Design review of the part built by this model. Coordinates are the model's own, in mm. Face numbers are marked on the shaded views. A direction names the side the tool comes from. Round coordinates to 2 decimals unless told otherwise and drop trailing zeros. Order: outer loops, then holes, each group sorted by start corner. A loop starts at its lowest first (then second) coordinate and runs counter-clockwise, first axis right, second up.
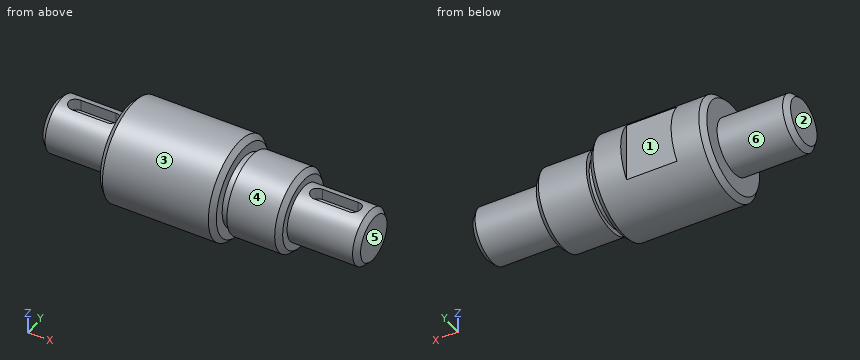
from build123d import *

# Parameters (mm, degrees)
SKETCH1_R               = 20
BOSS_EXTRUDE1_DEPTH     = 126
SKETCH2_OUTSIDE_W       = 69.624
SKETCH2_OUTSIDE_H       = 69.624
SKETCH2_OUTSIDE_R       = 11
CUT_EXTRUDE1_DEPTH      = 28
SKETCH3_OUTSIDE_W       = 69.624
SKETCH3_OUTSIDE_H       = 69.624
SKETCH3_OUTSIDE_R       = 11
CUT_EXTRUDE2_DEPTH      = 28
SKETCH4_OUTSIDE_W       = 69.624
SKETCH4_OUTSIDE_H       = 69.624
SKETCH4_OUTSIDE_R       = 16
CUT_EXTRUDE3_DEPTH      = 21
SKETCH5_OUTSIDE_W       = 69.624
SKETCH5_OUTSIDE_H       = 69.624
SKETCH5_OUTSIDE_R       = 14
CUT_EXTRUDE4_DEPTH      = 3
CHAMFER1_SIZE           = 2
CUT_EXTRUDE5_DEPTH      = 130.135587659
CUT_EXTRUDE5_DEPTH_BACK = 130.135587659
SKETCH6_W               = 20
SKETCH6_H               = 6
CUT_EXTRUDE6_DEPTH      = 5


with BuildPart() as part:
    # Sketch1 → Boss-Extrude1 (new body)
    with BuildSketch(Plane(origin=(0, 0, 0), x_dir=(0, 0, -1), z_dir=(1, 0, 0))):
        Circle(SKETCH1_R)
    extrude(amount=BOSS_EXTRUDE1_DEPTH)

    # Sketch2 outside → Cut-Extrude1 (cut)
    with BuildSketch(Plane.ZY):
        Rectangle(SKETCH2_OUTSIDE_W, SKETCH2_OUTSIDE_H)
        Circle(SKETCH2_OUTSIDE_R, mode=Mode.SUBTRACT)
    extrude(amount=-CUT_EXTRUDE1_DEPTH, mode=Mode.SUBTRACT)

    # Sketch3 outside → Cut-Extrude2 (cut)
    with BuildSketch(Plane(origin=(126, 0, 0), x_dir=(0, 0, -1), z_dir=(1, 0, 0))):
        Rectangle(SKETCH3_OUTSIDE_W, SKETCH3_OUTSIDE_H)
        with Locations(Location((0, 0, 0), (0, 0, 180))):
            Circle(SKETCH3_OUTSIDE_R, mode=Mode.SUBTRACT)
    extrude(amount=-CUT_EXTRUDE2_DEPTH, mode=Mode.SUBTRACT)

    # Sketch4 outside → Cut-Extrude3 (cut)
    with BuildSketch(Plane(origin=(98, 0, 0), x_dir=(0, 0, -1), z_dir=(1, 0, 0))):
        Rectangle(SKETCH4_OUTSIDE_W, SKETCH4_OUTSIDE_H)
        Circle(SKETCH4_OUTSIDE_R, mode=Mode.SUBTRACT)
    extrude(amount=-CUT_EXTRUDE3_DEPTH, mode=Mode.SUBTRACT)

    # Sketch5 outside → Cut-Extrude4 (cut)
    with BuildSketch(Plane(origin=(77, 0, 0), x_dir=(0, 0, -1), z_dir=(1, 0, 0))):
        Rectangle(SKETCH5_OUTSIDE_W, SKETCH5_OUTSIDE_H)
        Circle(SKETCH5_OUTSIDE_R, mode=Mode.SUBTRACT)
    extrude(amount=-CUT_EXTRUDE4_DEPTH, mode=Mode.SUBTRACT)

    # Chamfer1
    chamfer1_edges = [part.edges().sort_by_distance(p)[0] for p in [
        (0, 0, -11),
        (126, 0, -11),
        (98, 0, 16),
        (74, 0, 20),
        (28, 0, 20),
    ]]
    chamfer(chamfer1_edges, length=CHAMFER1_SIZE)

    # Sketch6 → Cut-Extrude5 (cut, two sides: drawn at the far end of the back side and taken through both)
    with BuildSketch(Plane.XY.offset(-CUT_EXTRUDE5_DEPTH_BACK)):
        with Locations((51, 19)):
            Rectangle(SKETCH6_W, SKETCH6_H)
    extrude(amount=CUT_EXTRUDE5_DEPTH + CUT_EXTRUDE5_DEPTH_BACK, mode=Mode.SUBTRACT)

    # Sketch7 → Cut-Extrude6 (cut)
    with BuildSketch(Plane.XY.offset(11)):
        with BuildLine():
            Line((8, 3), (22, 3))
            ThreePointArc((22, 3), (25, 0), (22, -3))
            Line((22, -3), (8, -3))
            ThreePointArc((8, -3), (5, 0), (8, 3))
        make_face()
        with BuildLine():
            Line((104, 3), (118, 3))
            ThreePointArc((118, 3), (121, 0), (118, -3))
            Line((118, -3), (104, -3))
            ThreePointArc((104, -3), (101, 0), (104, 3))
        make_face()
    extrude(amount=-CUT_EXTRUDE6_DEPTH, mode=Mode.SUBTRACT)


solid = part.part
1) To check wall thickness, follow line 1 along X through (y, z) = (-7, -9); line 2 along Y through (x, z) = (81, -0.5); line 3 along X through (y, z) = (17.5, 0). State the ranges of each line that lie inside material, in increasing order.
Results:
line 1: x = 28 to 98
line 2: y = -15.99 to 15.99
line 3: x = 28 to 41, 61 to 74
2) Take a section at C-C on x = 54. Give the boundary of the cut face in (y, z), plus the area to 3 significant figures.
Results:
outline: (16, -12) - (16, 12) arc R20 ccw (long way) to start
area: 1,190 mm2
3) The part is to be moulded in two halves that separate along X. For the marked faces 1, 2 and 3, say which applies: released by +X, released by -X, zero draft, split by the parting line, or undercut.
Results:
face 1: undercut
face 2: released by -X
face 3: zero draft
4) Clearance check with flat-ended pins moving along their axes: P1, Ø4.5, axis at y = 18.5, z = 1, coming from the +X side; P2, Ø5, axis at x = 111, z = 7, coming from the +Y side; P3, Ø2.5, axis at x = 11.5, z = 8, coming from the +Y side. State where each tip first meets the part, or that it passes through.
Results:
P1: stops at x = 74
P2: stops at y = 10.04
P3: stops at y = 8.69
5) Take a section at B-B on x = 67. Give the boundary of the cut face in (y, z), plus the area to 3 significant figures.
Results:
outline: circle Ø40 at (0, 0)
area: 1,260 mm2
6) For the marked faces 4, 5 and 6, list the 3-axis set-ups (+Z, -Z, +X, -X, +Y, -Y) from which the entire face can be reached by the end or side of a thin tool; tool diameter is ignored.
Results:
face 4: +X
face 5: +Z, -Z, +X, +Y, -Y
face 6: -X
